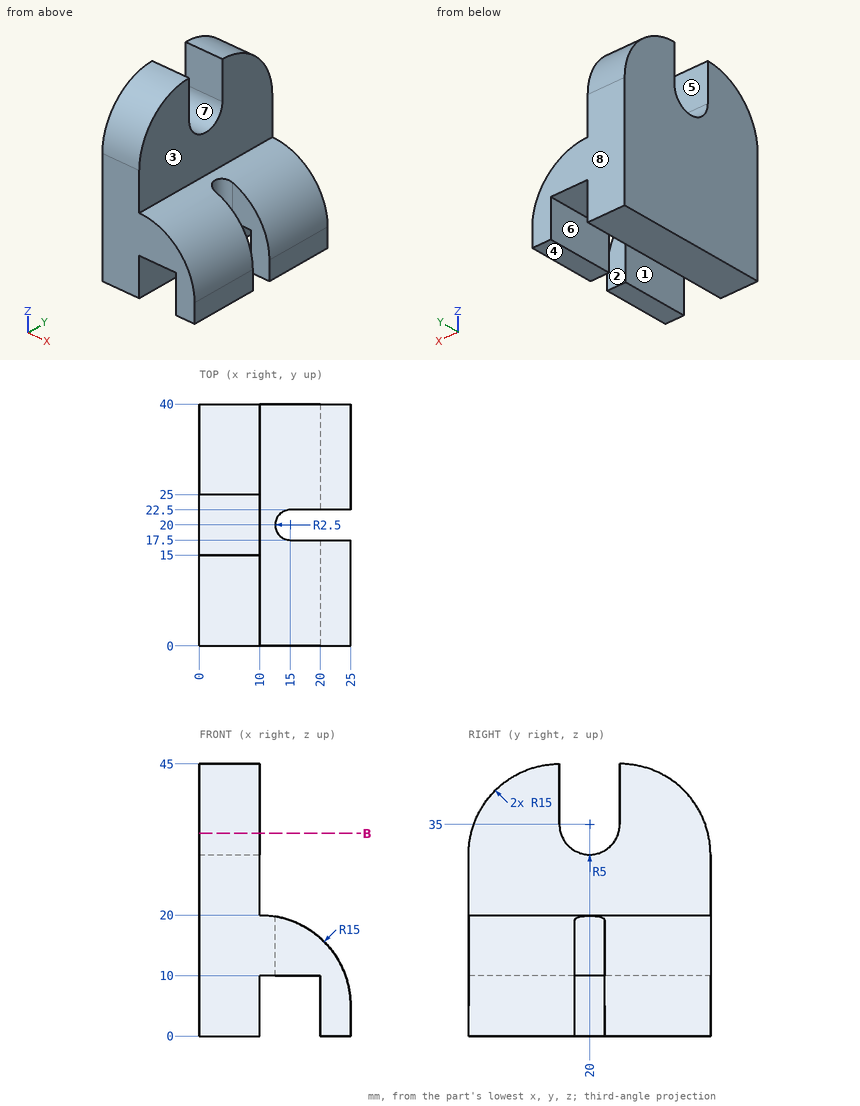
Could you check a few things on this drawing? It's one solid part, dimensions in mm from its lowest x, y, z. A direction names the side the tool comes from. Give positions to 0.01 mm unless a question says otherwise; leave off trailing zeros. Order: outer loops, then holes, each group sorted by start corner. A loop starts at its lowest first (then second) coordinate and runs counter-clockwise, first axis right, second up. Notation, with made-up numbers: (-19, -37) - (22, -37) arc R20 cw to (22, -28) - close; hole circle Ø10 at (38.25, 62). An arc over 180 degrees is marked (long way). Return JSON: item names as keys, results as strings. Group by question number.
Q1. Please list where these lines run through material, in increasing order: line 1 along Y through (x, z) = (4.75, 34); line 2 along X through (y, z) = (10.5, 5.5); line 3 along X through (y, z) = (2.5, 9.5). Write a range as [from, to].
Q2. Will these pins go through, and if not, where does the flat tip stop? pin 1 Ø2 at (x, y) = (12, 12) entering from -Z; pin 2 Ø8 at (x, z) = (4, 38.5) entering from +Y; pin 3 Ø8 at (x, z) = (3.5, 39.5) entering from -Y; pin 4 Ø12 at (x, z) = (19.5, 32) entering from +Y.
Q3. Which directions (+Z, -Z, +X, -X, +Y, -Y) give clear straight access to the entire face, cutting with the end or side of a thin tool? Please do the marked faces 1, 2, 3, 4 and 5.
Q4. Thinking about a two-plate mould opening in Y: for the marked faces 6, 7 and 8, which applies, pulls with the +Y half, pulls with the -Y half, needs draft (parallel to the pull), parting line crosses it, or undercut?
Q5. Suppose I cut it at B-B, the plane z = 33.5. Please give me the cut outline in (x, y), and give its area (3 significant figures).
Resolved:
{
 "1": {"line 1": "y = [0.54, 15.1], [24.9, 39.46]", "line 2": "x = [0, 10], [20, 24.99]", "line 3": "x = [0, 10], [20, 24.31]"},
 "2": {"pin 1": "stops at z = 10", "pin 2": "stops at y = 39.31", "pin 3": "stops at y = 1.04", "pin 4": "passes through"},
 "3": {"face 1": "-Z, +Y, -Y", "face 2": "+Z, -Z, +X", "face 3": "+Z, +X, +Y, -Y", "face 4": "-Z, +X, -X, +Y, -Y", "face 5": "+Z, +X, -X"},
 "4": {"face 6": "needs draft", "face 7": "undercut", "face 8": "pulls with the +Y half"},
 "5": {"outline": "(0, 0.41) - (10, 0.41) - (10, 15.23) - (0, 15.23) - close; (0, 24.77) - (10, 24.77) - (10, 39.59) - (0, 39.59) - close", "area": "296 mm2"}
}
